Autodesk Inventor part; units mm, degrees
ref_plane "YZ Plane" through (0, 0, 0) normal (1, 0, 0) x (0, 1, 0)
ref_plane "XZ Plane" through (0, 0, 0) normal (0, 1, 0) x (-1, 0, 0)
ref_plane "XY Plane" through (0, 0, 0) normal (0, 0, 1) x (1, 0, 0)
sketch "Sketch1" plane through (0, 0, 0) normal (0, 0, 1) x (1, 0, 0)
  circle A0 centre (0, 0) radius 19
  dimension "d0" = 38
extrude "Extrusion1" add sketch "Sketch1" along normal blind 30
ref_plane "Work Plane1" through (0, 0, 10) normal (0, 0, -1) x (-1, 0, 0)
sketch "Sketch2" plane through (0, 0, 10) normal (0, 0, -1) x (-1, 0, 0)
  circle A0 centre (0, 0) radius 30
  dimension "d4" = 60
extrude "Extrusion2" add sketch "Sketch2" against normal blind 10
sketch "Sketch3" plane through (0, 0, 30) normal (0, 0, 1) x (1, 0, 0)
  circle A0 centre (0, 0) radius 17.5
  dimension "d7" = 35
extrude "Extrusion3" add sketch "Sketch3" along normal blind 40
sketch "Sketch4" plane through (0, 0, 70) normal (0, 0, 1) x (1, 0, 0)
  circle A0 centre (0, 0) radius 15
  dimension "d10" = 30
extrude "Extrusion4" add sketch "Sketch4" along normal blind 85
sketch "Sketch5" plane through (0, 0, 155) normal (0, 0, 1) x (1, 0, 0)
  line L0 (-3, 11.6969) -> (-3, 14.6969)
  circle A0 centre (0, 0) radius 15
  line L1 (3, 11.6969) -> (3, 14.6969)
  arc A1 (3, 14.6969) -> (-3, 14.6969) centre (0, 0) ccw
  line L2 (-3, 14.6969) -> (-3, 11.6969)
  line L3 (-3, 11.6969) -> (3, 11.6969)
  line L4 (3, 11.6969) -> (3, 14.6969)
  dimension "d15" = 3
  dimension "d16" = 6
extrude "Extrusion5" cut sketch "Sketch5" against normal blind 85 contours L0 A0 L1 L3 picked at (0.3353, 12.7867)
properties part number "project handle part"
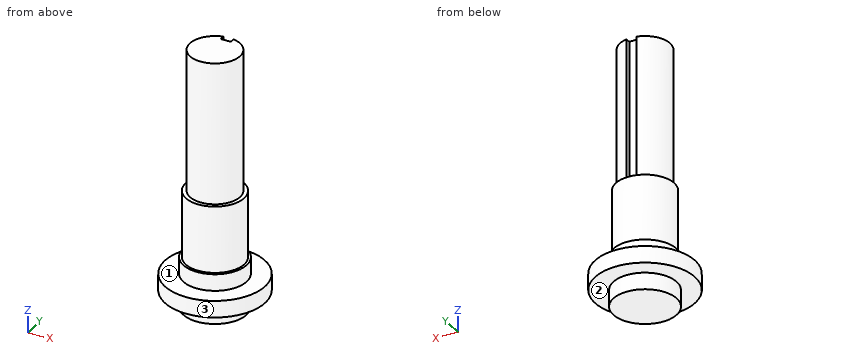
Here's how the part is built. I have some questions about the finished solid (model axes, mm). Face numbers are marked on the shaded views. A direction names the side the tool comes from. Coordinates: 2 decimals unless noted, no trailing zeros. Order: outer loops, then holes, each group sorted by start corner. A loop starts at its lowest first (then second) coordinate and runs counter-clockwise, first axis right, second up.
1) Imagine slicing it at D-D on z = 129. List the corners of the cut face in (x, y) for me.
2) Will these pins go through, and if not, where does the flat tip stop? pin 1 (1.5 mm diameter, centred on x = -6.5, y = 15, fed in from +Z); pin 2 (1 mm diameter, centred on x = -9.5, y = 20.5, fed in from +Z); pin 3 (10 mm diameter, centred on y = 6.5, z = 60, fed in from +X); pin 4 (18 mm diameter, centred on x = 3.5, y = 4, fed in from -Z).
3) Imagine slicing it at C-C on z = 62. List the corners of the cut face in (x, y) for me.
4) Imagine slicing it at B-B on x = 0. List the corners of the cut face in (y, z) for me, and give its area (3 significant figures).
5) Which directions (+Z, -Z, +X, -X, +Y, -Y) give clear straight access to the entire face, cutting with the end or side of a thin tool? Please do the marked faces 1, 2 and 3.
6) I need wall thicknesses on line 1 (Z direction, x = -7, y = 16); line 2 (Z direction, x = -23, y = -0.5); line 3 (Y direction, x = -9, z = 57). Which ranges of each line are inside material? Lowest first, please.
7) Imagine slicing it at A-A on y = 0. List the corners of the cut face in (x, z) for me, and give its area (3 significant figures).
Response values:
1. outline: (-3, 11.7) - (-3, 14.7) arc R15 ccw (long way) to (3, 14.7) - (3, 11.7) - close
2. pin 1: stops at z = 70
2. pin 2: stops at z = 20
2. pin 3: stops at x = 17.44
2. pin 4: stops at z = 0
3. outline: circle Ø35 at (0, 0)
4. outline: (-30, 10) - (-19, 10) - (-19, 0) - (19, 0) - (19, 10) - (30, 10) - (30, 20) - (19, 20) - (19, 30) - (17.5, 30) - (17.5, 70) - (11.7, 70) - (11.7, 155) - (-15, 155) - (-15, 70) - (-17.5, 70) - (-17.5, 30) - (-19, 30) - (-19, 20) - (-30, 20) - close
4. area: 5,030 mm2
5. face 1: +Z
5. face 2: -Z
5. face 3: +Z, -Z
6. line 1: z = 0 to 70
6. line 2: z = 10 to 20
6. line 3: y = -15.01 to 15.01
7. outline: (-30, 10) - (-19, 10) - (-19, 0) - (19, 0) - (19, 10) - (30, 10) - (30, 20) - (19, 20) - (19, 30) - (17.5, 30) - (17.5, 70) - (15, 70) - (15, 155) - (-15, 155) - (-15, 70) - (-17.5, 70) - (-17.5, 30) - (-19, 30) - (-19, 20) - (-30, 20) - close
7. area: 5,310 mm2
